```python
from build123d import *

# Parameters (mm, degrees)
SKETCH1_W             = 32
SKETCH1_H             = 62
BOSS_EXTRUDE4_DEPTH   = 2
SKETCH2_W             = 32
SKETCH2_H             = 62
SKETCH2_W_2           = 28
SKETCH2_H_2           = 58
BOSS_EXTRUDE5_DEPTH   = 18
SKETCH3_R             = 2.1
CUT_EXTRUDE1_DEPTH    = 10
SKETCH5_W             = 10.2
SKETCH5_H             = 4.7
CUT_EXTRUDE2_DEPTH    = 2
FILLET13_R            = 2
FILLET14_R            = 4
FILLET15_R            = 1
BODY_MOVE_COPY1_ANGLE = 180


with BuildPart() as part:
    # Sketch1 → Boss-Extrude4 (new body)
    with BuildSketch(Plane.XY):
        Rectangle(SKETCH1_W, SKETCH1_H)
    extrude(amount=BOSS_EXTRUDE4_DEPTH)

    # Sketch2 → Boss-Extrude5 (add)
    with BuildSketch(Plane.XY):
        Rectangle(SKETCH2_W, SKETCH2_H)
        Rectangle(SKETCH2_W_2, SKETCH2_H_2, mode=Mode.SUBTRACT)
    extrude(amount=-BOSS_EXTRUDE5_DEPTH)

    # Sketch3 → Cut-Extrude1 (cut)
    with BuildSketch(Plane(origin=(0, 31, 0), x_dir=(1, 0, 0), z_dir=(0, 1, 0))):
        with Locations(Location((-9, 6.5, 0), (0, 0, 270))):
            Circle(SKETCH3_R)
        with Locations(Location((9, 6.5, 0), (0, 0, 270))):
            Circle(SKETCH3_R)
    extrude(amount=-CUT_EXTRUDE1_DEPTH, mode=Mode.SUBTRACT)

    # Sketch5 → Cut-Extrude2 (cut)
    with BuildSketch(Plane.XZ.offset(31)):
        with Locations((0, -15.65)):
            Rectangle(SKETCH5_W, SKETCH5_H)
    extrude(amount=-CUT_EXTRUDE2_DEPTH, mode=Mode.SUBTRACT)

    # Fillet13
    fillet13_edges = [part.edges().sort_by_distance(p)[0] for p in [
        (14, 29, -9),
        (-14, 29, -9),
        (-14, -29, -9),
        (14, -29, -9),
        (-5.1, -30, -13.3),
        (5.1, -30, -13.3),
    ]]
    fillet(fillet13_edges, radius=FILLET13_R)

    # Fillet14
    fillet14_edges = [part.edges().sort_by_distance(p)[0] for p in [
        (16, -31, -8),
        (-16, -31, -8),
        (-16, 31, -8),
        (16, 31, -8),
    ]]
    fillet(fillet14_edges, radius=FILLET14_R)

    # Fillet15
    fillet15_edges = [part.edges().sort_by_distance(p)[0] for p in [
        (16, 0, 2),
        (0, -31, 2),
        (0, 31, 2),
        (-16, 0, 2),
        (-14.828427125, -29.828427125, 2),
        (-14.828427125, 29.828427125, 2),
        (14.828427125, 29.828427125, 2),
        (14.828427125, -29.828427125, 2),
        (-9, 31, -8.6),
        (9, 31, -8.6),
        (5.1, -31, -16.65),
        (-5.1, -31, -16.65),
        (0, -31, -13.3),
        (-4.514213562, -31, -13.885786438),
        (4.514213562, -31, -13.885786438),
    ]]
    fillet(fillet15_edges, radius=FILLET15_R)


with BuildPart() as part_1:
    # Body-Move/Copy1: moved
    add(part.part.rotate(Axis((0, 0, -8), (0, 1, 0)), BODY_MOVE_COPY1_ANGLE))


solid = part_1.part
```
The model under review builds one solid part; all positions refer to its coordinate system, in mm. A direction names the side the tool comes from. Round coordinates to 2 decimals unless told otherwise and drop trailing zeros. Order: outer loops, then holes, each group sorted by start corner. A loop starts at its lowest first (then second) coordinate and runs counter-clockwise, first axis right, second up. Notation, with made-up numbers: (81.25, 45) -> (101.25, 45) arc R29 cw to (101.25, 76) -> close; hole circle Ø10 at (-31, 51.5). An arc over 180 degrees is marked (long way). One line per item, written item: value. Start each with the question number.
Q1. Machinability: for faces 1 (the face through (4.5, -29.49, -2.13)), 2 (the face through (13.4, 28.43, -6.87)), 3 (the face through (7.581, 29.507, -7.952)), 4 (the face through (-14.859, 29.797, -7.367)), which of the approach directions +Z, -Z, +X, -X, +Y, -Y give a long, thin tool a straight path to every point of the face, cutting with its end or side? Answer none if there is none.
Q2. Wall thickness on line 1 (X direction, y = 7, z = -15.25); line 2 (Y direction, x = 6, z = -0.75); line 3 (X direction, y = 29.7, z = -9.5): over which ranges is each line inside the solid? List them lowest first.
Q3. Clearance check with flat-ended pins moving along their axes: pin 1 Ø5 at (x, z) = (-9, -9.5) entering from +Y; pin 2 Ø4 at (x, y) = (11, 2.5) entering from +Z; pin 3 Ø1.1 at (y, z) = (-29.5, 0.5) entering from +X. State where each tip first meets the part, or that it passes through.
Q4. Take a section at A-A (x = 9). Write out the cut boundary in (y, z), and give its area (3 significant figures).
Q5. Take a section at B-B (y = -7). Write out the cut boundary in (x, z), and give its area (3 significant figures).
Q6. Mouldability with a two-part tool opening along X and no side actions: class faces 5 (the face through (16, 0, -8)), 6 (the face through (13.4, -28.43, -6.87)), 7 (the face through (0, -31, -10)), 8 (the face through (14, 0, -7)) as released by +X, released by -X, zero draft, split by the parting line, or undercut.
Reported:
1. face 1: +Z, -Y
1. face 2: +Z
1. face 3: +Y
1. face 4: +Z, -Z, -X, +Y
2. line 1: x = -16 to -14, 14 to 16
2. line 2: y = -31 to -29, 29 to 31
2. line 3: x = -14.95 to -11.1, -6.9 to 6.9, 11.1 to 14.95
3. pin 1: stops at y = 30.8
3. pin 2: stops at z = -16
3. pin 3: stops at x = 15.49
4. outline: (-31, -17) arc R1 ccw to (-30, -18) -> (30, -18) arc R1 ccw to (31, -17) -> (31, -12.6) arc R1 ccw to (30, -11.6) -> (29, -11.6) -> (29, -16) -> (-29, -16) -> (-29, 2) -> (-31, 2) -> close; (29, -7.4) -> (30, -7.4) arc R1 ccw to (31, -6.4) -> (31, 2) -> (29, 2) -> close
4. area: 187 mm2
5. outline: (-16, -17) arc R1 ccw to (-15, -18) -> (15, -18) arc R1 ccw to (16, -17) -> (16, 2) -> (14, 2) -> (14, -16) -> (-14, -16) -> (-14, 2) -> (-16, 2) -> close
5. area: 136 mm2
6. face 5: released by +X
6. face 6: undercut
6. face 7: zero draft
6. face 8: undercut
